Can you work these out from the model? Positions are in its coordinate system, mm. A direction names the side the tool comes from. Round coordinates to 2 decimals unless told otherwise and drop trailing zeros. Write each loop counter-clockwise with the first axis right and the second up, starting at its lowest first coordinate (ties: lowest second). Pieces come first, ordered by that corner, then holes.
Q1. If we section it at B-B (z = 6): Please give me the cut outline in (x, y) (3 decimals).
Q2. I'm going to push flat-ended pins straight in: pin 1 Ø4 at (y, z) = (55.5, 7) entering from -X; pin 2 Ø10 at (x, y) = (-36, 50) entering from -Z; pin 3 Ø4 at (x, z) = (54, 7.5) entering from +Y. Where does each tip first touch, or does it pass through?
Q3. If we section it at A-A (y = -11): Please give me the cut outline in (x, z).
Q4. Please list where these lines run through material, in increasing order: line 1 along X through (y, z) = (-19, 11.5); line 2 along X through (y, z) = (37, 11); line 3 along X through (y, z) = (-28, 10.25).
Q5. If we section it at D-D (y = -43): Please give me the cut outline in (x, z).
Q6. If we section it at C-C (x = 0): Please give me the cut outline in (y, z) (3 decimals), plus the area to 3 significant figures.
Q7. We'd pull the mould along X, two halves only. Please class faces 4 (the cylindrical face through (73.361, 63.255, 6.261)), 5 (the cylindrical face through (-33.836, 52.361, 6.261)), 6 (the flat face through (-1, -28, 0)): +X half, -X half, draft (parallel to the pull), parting line (faces both ways), or undercut.
Q8. For faces 1 (the flat face through (50, 71.02, 6)), 2 (the flat face through (-37.18, 66.04, 6.26)), 3 (the flat face through (0, -69.85, 6)), which set-ups out of +Z, -Z, +X, -X, +Y, -Y let a thin tool reach every point of the face, with its end or its side?
Autodesk Inventor part; units mm, degrees
ref_plane "YZ Plane" through (0, 0, 0) normal (1, 0, 0) x (0, 1, 0)
ref_plane "XZ Plane" through (0, 0, 0) normal (0, 1, 0) x (-1, 0, 0)
ref_plane "XY Plane" through (0, 0, 0) normal (0, 0, 1) x (1, 0, 0)
sketch "Sketch1" plane through (0, 0, 0) normal (0, 0, 1) x (1, 0, 0)
  arc A0 (-22.225, 0) -> (22.225, 0) centre (0, 0) ccw
  arc A1 (34.925, -69.85) -> (50.8, -53.975) centre (34.925, -53.975) ccw
  arc A2 (-50.8, -53.975) -> (-34.925, -69.85) centre (-34.925, -53.975) ccw
  line L0 (-34.925, -69.85) -> (34.925, -69.85)
  line L1 (-50.8, -53.975) -> (-78.105, 49.53)
  line L2 (50.8, -53.975) -> (78.105, 49.53)
  line L3 (-33.655, 49.53) -> (-22.225, 0)
  line L4 (33.655, 49.53) -> (22.225, 0)
  line L5 (-61.5491, 71.0198) -> (-39.9288, 76.7156)
  line L6 (-39.9288, 76.7156) -> (-34.3567, 55.0708)
  line L7 (61.5491, 71.0198) -> (38.6142, 71.0198)
  line L8 (38.6142, 71.0198) -> (32.2206, 43.3143)
  arc A3 (-33.655, 49.53) -> (-34.3567, 55.0708) centre (-55.88, 49.53) ccw
  arc A4 (-61.5347, 71.0236) -> (-75.2129, 38.5669) centre (-55.88, 49.53) ccw
  arc A5 (75.2129, 38.5669) -> (50.2109, 71.0198) centre (55.88, 49.53) ccw
  arc A6 (35.9025, 59.269) -> (33.655, 49.53) centre (55.88, 49.53) ccw
  dimension "d1" = 31.75
  dimension "d5" = 31.75
  dimension "d8" = 34.925
  dimension "d11" = 69.85
  dimension "d15" = 119.38
  dimension "d16" = 55.88
extrude "Extrusion1" add sketch "Sketch1" along normal blind 12.7 contours A0 L4 L8 L7 A5 L2 A1 L0 A2 L1 A4 L5 L6 A3 L3
properties part number "4-2"
A:
1. outline: (-78.105, 49.53) - (-50.8, -53.975) arc R15.875 ccw to (-34.925, -69.85) - (34.925, -69.85) arc R15.875 ccw to (50.8, -53.975) - (78.105, 49.53) arc R22.225 ccw to (61.549, 71.02) - (38.614, 71.02) - (33.655, 49.53) - (22.225, 0) arc R22.225 cw to (-22.225, 0) - (-33.655, 49.53) arc R22.228 ccw to (-34.357, 55.071) - (-39.929, 76.716) - (-61.549, 71.02) arc R22.225 ccw to start
2. pin 1: stops at x = -77.75
2. pin 2: stops at z = 0
2. pin 3: stops at y = 71.02
3. outline: (-62.14, 0) - (-19.31, 0) - (-19.31, 12.7) - (-62.14, 12.7) - close; (19.31, 0) - (62.14, 0) - (62.14, 12.7) - (19.31, 12.7) - close
4. line 1: x = -60.03 to -11.53, 11.53 to 60.03
4. line 2: x = -74.8 to -30.76, 30.76 to 74.8
4. line 3: x = -57.65 to 57.65
5. outline: (-53.7, 0) - (53.7, 0) - (53.7, 12.7) - (-53.7, 12.7) - close
6. outline: (-69.85, 0) - (-22.225, 0) - (-22.225, 12.7) - (-69.85, 12.7) - close
6. area: 605 mm2
7. face 4: +X half
7. face 5: undercut
7. face 6: draft
8. face 1: +Z, -Z, +X, +Y
8. face 2: +Z, -Z, +Y
8. face 3: +Z, -Z, +X, -X, -Y
